Drawing for the job (mm, zero at the part's lowest x, y, z). Give positions to 0.01 mm unless a question says otherwise; leave off trailing zeros. Loops run counter-clockwise (first coordinate to the right, second up) from the corner with the lowest first, then second, coordinate; pieces in that order, holes last. Notation, with made-up numbers: M 45.25,-3 L 59.25,-3 A20 ccw 59.25,20 Z; hole C 82.25,67.25 d7. An arc over 180 degrees is marked long. Use CSV: the item, a comma, the result in double quotes. Start each with the question number.
(1) Wall check: line 1 along X through (y, z) = (4.6, 103.5); line 2 along X through (y, z) = (2.5, 40). Give the ranges that are in metal, low to high. Write a range as from..to.
(2) Flat gauge pin, fed straight in: P1, Ø16.5, axis at x = 25.5, z = 35, coming from the +Y side. Where does the tip first touch, or does it go through?
(3) Slice it at B-B on z = 93. List the corners of the cut face in (x, y).
(4) Slice it at C-C on x = 72. List the corners of the cut face in (y, z).
(5) Two-plate mould, pull along Z, no slides. Class the marked faces 1 and 2: pulls with the +Z half, pulls with the -Z half, needs draft (parallel to the pull), parting line crosses it, or undercut.
(6) Slice it at A-A on y = 4.2. List the corners of the cut face in (x, z), and give its area (3 significant figures).
(7) Slice it at D-D on z = 53.5. List the corners of the cut face in (x, y).
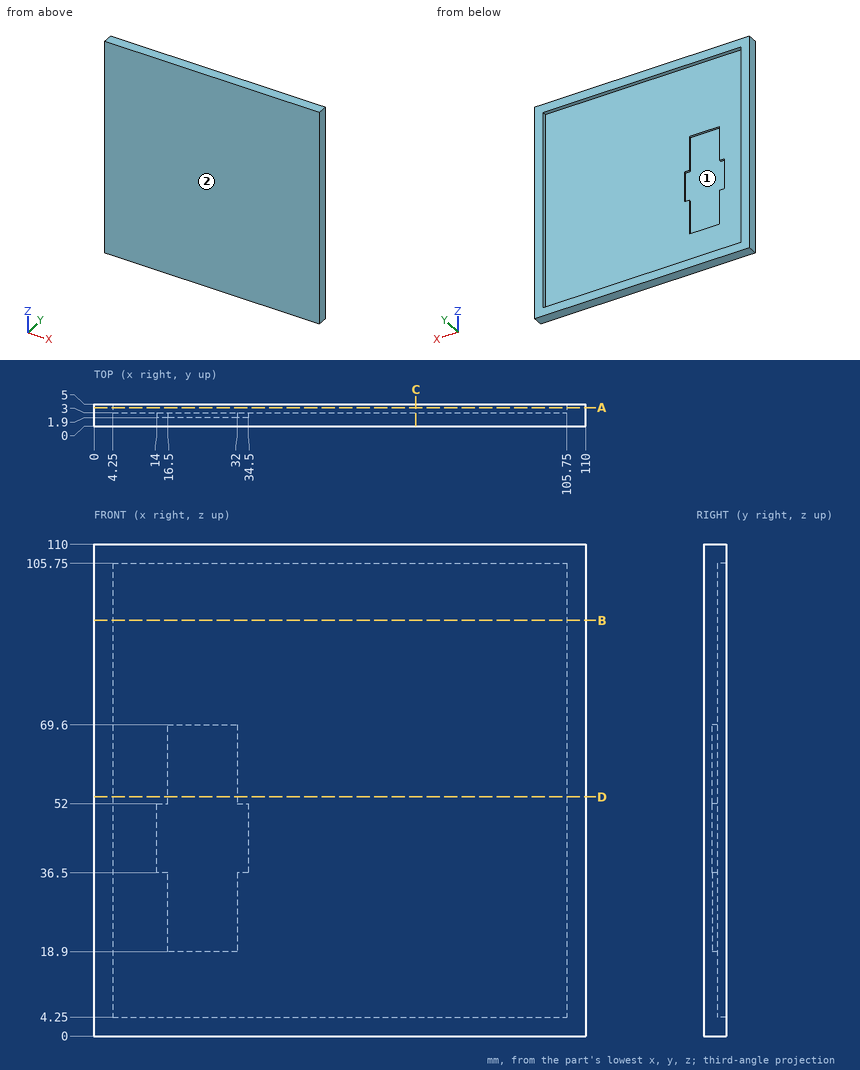
Reply:
1,line 1,"x = 0..4.25, 105.75..110"
1,line 2,"x = 0..14, 34.5..110"
2,P1,"stops at y = 3"
3,outline,"M 0,0 L 110,0 L 110,5 L 105.75,5 L 105.75,3 L 4.25,3 L 4.25,5 L 0,5 Z"
4,outline,"M 0,0 L 5,0 L 5,4.25 L 3,4.25 L 3,105.75 L 5,105.75 L 5,110 L 0,110 Z"
5,face 1,"undercut"
5,face 2,"needs draft"
6,outline,"M 0,0 L 110,0 L 110,110 L 0,110 Z; hole M 4.25,4.25 L 105.75,4.25 L 105.75,105.75 L 4.25,105.75 Z"
6,area,"1,800 mm^2"
7,outline,"M 0,0 L 110,0 L 110,5 L 105.75,5 L 105.75,3 L 32,3 L 32,1.9 L 16.5,1.9 L 16.5,3 L 4.25,3 L 4.25,5 L 0,5 Z"
